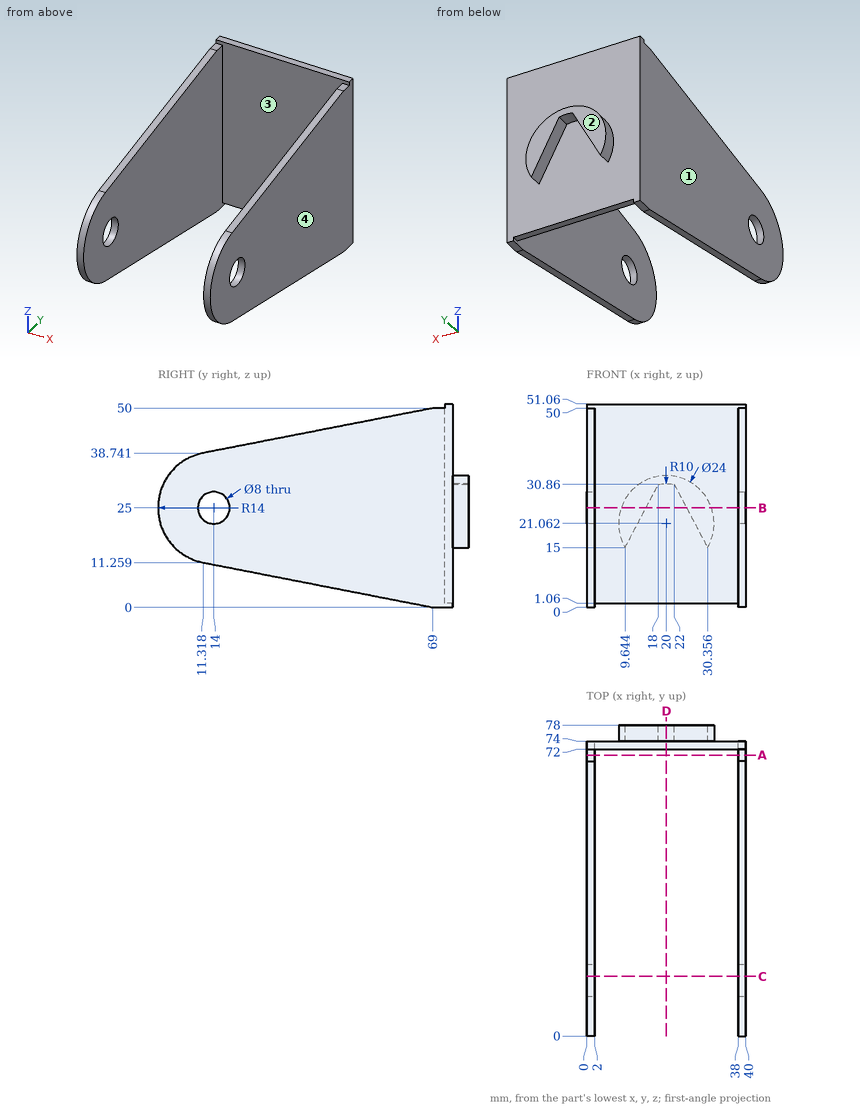
Study the drawing (mm; zero at the part's minimum x, y, z) and answer. Coordinates: 2 decimals unless noted, no trailing zeros. Loops run counter-clockwise (first coordinate to the right, second up) from the corner with the lowest first, then second, coordinate; pieces in that order, holes last. Notation, with made-up numbers: M -10,38 L 14,38 A6 ccw 14,45 Z; hole C -3.5,27 d9. An arc over 180 degrees is marked long. Answer as a JSON object with one key per item and string values. Group by question number.
Item 1: Section C-C (y = 15) is taken. Write down the section's boundary in (x, z).
Item 2: Consider L1, parallel to Y at x = 39, z = 25; L2, parallel to X at y = 60, z = 2.5; L3, parallel to Y at x = 15, z = 44.5. Determine where each line is inside the solid, lowest interval first.
Item 3: Each of these flat-tipped pins is pushed along its axis until it touches: P1, Ø6, axis at x = 32, z = 19.5, coming from the -Y side; P2, Ø10, axis at x = 17, z = 40.5, coming from the +Y side; P3, Ø1.6, axis at x = 23, y = 73, coming from the -Z side. Where does it stop, or does it pass through?
Item 4: Section D-D (x = 20) is taken. Write down the section's boundary in (y, z), and give its area (3 significant figures).
Item 5: Section A-A (y = 70.5) is taken. Write down the section's boundary in (x, z), and give its area (3 significant figures).
Item 6: Section B-B (z = 25) is taken. Write down the section's boundary in (x, y) (1 decimal), and give its area (3 significant figures).
Item 7: Determine the mould class of the marked faces 1, 2, 3 and 4 for opening direction X: +X half, -X half, draft (parallel to the pull), parting line (faces both ways), or undercut.
Solved:
{
 "1": {"outline": "M 0,10.54 L 2,10.54 L 2,21.13 L 0,21.13 Z; M 0,28.87 L 2,28.87 L 2,39.46 L 0,39.46 Z; M 38,10.54 L 40,10.54 L 40,21.13 L 38,21.13 Z; M 38,28.87 L 40,28.87 L 40,39.46 L 38,39.46 Z"},
 "2": {"L1": "y = 0 to 10, 18 to 74", "L2": "x = 0 to 2, 38 to 40", "L3": "y = 72 to 74"},
 "3": {"P1": "stops at y = 72", "P2": "stops at y = 74", "P3": "stops at z = 1.06"},
 "4": {"outline": "M 72,1.06 L 74,1.06 L 74,31.06 L 78,31.06 L 78,33.06 L 74,33.06 L 74,51.06 L 72,51.06 Z", "area": "108 mm2"},
 "5": {"outline": "M 0,0 L 2,0 L 2,50 L 0,50 Z; M 38,0 L 40,0 L 40,50 L 38,50 Z", "area": "200 mm2"},
 "6": {"outline": "M 0,0 L 2,0 L 2,10 L 0,10 Z; M 0,18 L 2,18 L 2,72 L 38,72 L 38,18 L 40,18 L 40,74 L 31.3,74 L 31.3,78 L 25.1,78 L 25.1,74 L 14.9,74 L 14.9,78 L 8.7,78 L 8.7,74 L 0,74 Z; M 38,0 L 40,0 L 40,10 L 38,10 Z", "area": "386 mm2"},
 "7": {"face 1": "-X half", "face 2": "draft", "face 3": "undercut", "face 4": "+X half"}
}
